from build123d import *

# Parameters (mm, degrees)
SKETCH1_W           = 39.4
SKETCH1_H           = 41.6
BOSS_EXTRUDE1_DEPTH = 16.1
SKETCH1_3_W         = 44
SKETCH1_3_H         = 45.6
SKETCH1_3_W_2       = 39.4
SKETCH1_3_H_2       = 41.6
BOSS_EXTRUDE2_DEPTH = 6.1
SKETCH2_R           = 2
CUT_EXTRUDE1_DEPTH  = 17.1


with BuildPart() as part:
    # Sketch1 → Boss-Extrude1 (new body)
    with BuildSketch(Plane.XY):
        with Locations((-4.36, -1.18)):
            Rectangle(SKETCH1_W, SKETCH1_H)
    extrude(amount=BOSS_EXTRUDE1_DEPTH)

    # Sketch1<3> → Boss-Extrude2 (add)
    with BuildSketch(Plane.XY):
        with Locations((-4.34, -0.9)):
            Rectangle(SKETCH1_3_W, SKETCH1_3_H)
        with Locations((-4.36, -1.18)):
            Rectangle(SKETCH1_3_W_2, SKETCH1_3_H_2, mode=Mode.SUBTRACT)
    extrude(amount=BOSS_EXTRUDE2_DEPTH)

    # Sketch2 → Cut-Extrude1 (cut, through all)
    with BuildSketch(Plane.XY.offset(16.1)):
        with Locations((-20.623955183, -18.125224269)):
            Circle(SKETCH2_R)
        with Locations((-20.623955183, 16.074219179)):
            Circle(SKETCH2_R)
        with Locations((11.253691187, 16.074219179)):
            Circle(SKETCH2_R)
        with Locations((11.253691187, -18.125224269)):
            Circle(SKETCH2_R)
    extrude(amount=-CUT_EXTRUDE1_DEPTH, mode=Mode.SUBTRACT)


solid = part.part
The listing builds one solid part. Answer for the finished solid, in the listing's coordinates (mm). A direction names the side the tool comes from. Round coordinates to 2 decimals unless told otherwise and drop trailing zeros. Order: outer loops, then holes, each group sorted by start corner. A loop starts at its lowest first (then second) coordinate and runs counter-clockwise, first axis right, second up. Notation, with made-up numbers: M 84.5,72 L 107.5,72 A19 ccw 107.5,88 Z; hole C 80.5,41.5 d10. An arc over 180 degrees is marked long. Answer in a Markdown table with one row per item. Add a question column.
1) Which of the six approach directions +Z, -Z, +X, -X, +Y, -Y give full straight-line access (tool end or side, diameter ignored) to faces 1 (the face through (-5, -21.98, 11)), 2 (the face through (15.34, -1, 11)), 3 (the face through (-26, -1, 6.1)), 4 (the face through (-5, -23.7, 3)), 5 (the face through (-5, -1, 16.1))?
2) The part is cut by section D-D on x = -21. Determine the outline of the cut face in (y, z), plus the area to 3 significant figures.
3) Consider line 1 along X through (y, z) = (-18, 12.25); line 2 along Y through (x, z) = (-21.5, 5.5); line 3 along Y through (x, z) = (0, 11.5). Determine where each line is inside the solid, lowest interval first. Write a range as from..to.
4) Flat-ended cylindrical pins translate along their axes: pin 1 Ø8 at (y, z) = (-5, 12) entering from -X; pin 2 Ø5 at (y, z) = (1, 10.5) entering from +X; pin 3 Ø6.5 at (x, y) = (-20.62, 16.07) entering from -Z; pin 4 Ø3.5 at (x, y) = (11.25, 16.07) entering from +Z. Find the tip coordinate at first contact, or state that the pin passes through.
5) The part is cut by section A-A on x = -3. Determine the outline of the cut face in (y, z).
6) The part is cut by section C-C on y = -8. Determine the outline of the cut face in (x, z), plus the area to 3 significant figures.
7) The part is cut by section B-B on z = 15. Determine the outline of the cut face in (x, y).
8) Determine the mould class of faces 6 (the face through (-24.06, -1, 11)), 7 (the face through (-19.55, 17.76, 8.16)), 8 (the face through (-5, 19.62, 11)) for opening direction Y: pulls with the +Y half, pulls with the -Y half, needs draft (parallel to the pull), parting line crosses it, or undercut.
Findings below:
| question | item | result |
|---|---|---|
| 1 | face 1 | +Z, +X, -X, -Y |
| 1 | face 2 | +Z, +X, +Y, -Y |
| 1 | face 3 | +Z |
| 1 | face 4 | +Z, -Z, +X, -X, -Y |
| 1 | face 5 | +Z, +X, -X, +Y, -Y |
| 2 | outline | M -23.7,0 L -20.09,0 L -20.09,16.1 L -21.98,16.1 L -21.98,6.1 L -23.7,6.1 Z; M -16.16,0 L 14.11,0 L 14.11,16.1 L -16.16,16.1 Z; M 18.04,0 L 21.9,0 L 21.9,6.1 L 19.62,6.1 L 19.62,16.1 L 18.04,16.1 Z |
| 2 | area | 568 mm² |
| 3 | line 1 | x = -24.06..-22.62, -18.63..9.26, 13.25..15.34 |
| 3 | line 2 | y = -23.7..-19.92, -16.33..14.28, 17.87..21.9 |
| 3 | line 3 | y = -21.98..19.62 |
| 4 | pin 1 | stops at x = -24.06 |
| 4 | pin 2 | stops at x = 15.34 |
| 4 | pin 3 | stops at z = 0 |
| 4 | pin 4 | passes through |
| 5 | outline | M -23.7,0 L 21.9,0 L 21.9,6.1 L 19.62,6.1 L 19.62,16.1 L -21.98,16.1 L -21.98,6.1 L -23.7,6.1 Z |
| 6 | outline | M -26.34,0 L 17.66,0 L 17.66,6.1 L 15.34,6.1 L 15.34,16.1 L -24.06,16.1 L -24.06,6.1 L -26.34,6.1 Z |
| 6 | area | 662 mm² |
| 7 | outline | M -24.06,-21.98 L 15.34,-21.98 L 15.34,19.62 L -24.06,19.62 Z; hole C -20.62,-18.13 d4; hole C -20.62,16.07 d4; hole C 11.25,-18.13 d4; hole C 11.25,16.07 d4 |
| 8 | face 6 | needs draft |
| 8 | face 7 | undercut |
| 8 | face 8 | pulls with the +Y half |
